Autodesk Inventor part; units mm, degrees
ref_plane "YZ Plane" through (0, 0, 0) normal (1, 0, 0) x (0, 1, 0)
ref_plane "XZ Plane" through (0, 0, 0) normal (0, 1, 0) x (-1, 0, 0)
ref_plane "XY Plane" through (0, 0, 0) normal (0, 0, 1) x (1, 0, 0)
sketch "草圖1" plane through (0, 0, 0) normal (0, 0, 1) x (1, 0, 0)
  circle A0 centre (0, 0) radius 17.5
  circle A1 centre (120, 0) radius 17.5
  line L0 (0, 17.5) -> (120, 17.5)
  line L1 (120, 17.5) -> (120, -17.5)
  line L2 (120, -17.5) -> (0, -17.5)
  line L3 (0, -17.5) -> (0, 17.5)
  dimension "d0" = 35
  dimension "d1" = 35
  dimension "d4" = 120
  dimension "d5" = 35
extrude "擠出1" add sketch "草圖1" along normal blind 15
sketch "草圖2" plane through (0, 0, 15) normal (0, 0, 1) x (1, 0, 0)
  circle A0 centre (0, 0) radius 14
  arc A1 (120, -17.5) -> (120, 17.5) centre (120, 0) ccw
  circle A2 centre (120, 0) radius 14
  dimension "d6" = 28
  dimension "d7" = 28
extrude "擠出2" cut sketch "草圖2" against normal blind 10
sketch "草圖3" plane through (0, 0, 0) normal (1, 0, 0) x (0, 1, 0)
  circle A0 centre (0, -33.7441) radius 48.7441
  point P0 (0, 0)
extrude "擠出3" cut sketch "草圖3" along normal through all both and the other way through all keep common part
sketch "草圖5" plane through (0, 0, 0) normal (0, 0, -1) x (-1, 0, 0)
  circle A0 centre (0, 0) radius 14
  line L0 (0, 17.5) -> (-120, 17.5)
  arc A1 (-120, 17.5) -> (-120, -17.5) centre (-120, 0) ccw
  line L1 (-120, -17.5) -> (0, -17.5)
  arc A2 (0, -17.5) -> (0, 17.5) centre (0, 0) ccw
  line L2 (0, 17.5) -> (-120, 17.5)
  line L3 (-87.5, 17.5) -> (-87.5, -17.5)
  line L4 (-120, -17.5) -> (0, -17.5)
  dimension "d13" = 50
extrude "擠出4" add sketch "草圖5" along normal blind 20 contours A0 | A2 L1 L3 L0
properties part number "第一臂"
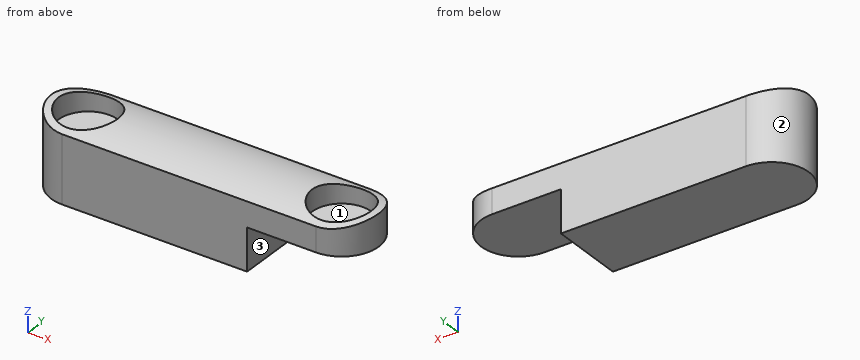
Design review of the part built by this model. Coordinates are the model's own, in mm. Face numbers are marked on the shaded views. A direction names the side the tool comes from. Round coordinates to 2 decimals unless told otherwise and drop trailing zeros. Write each loop counter-clockwise with the first axis right and the second up, starting at its lowest first coordinate (ties: lowest second). Pieces come first, ordered by that corner, then holes.
Item 1: Consider section C-C on x = 113. Give the boundary of the cut face in (y, z).
Item 2: Consider section A-A on z = 7.5. Give the boundary of the cut face in (x, y).
Item 3: For the marked faces 1, 2 and 3, list the 3-axis set-ups (+Z, -Z, +X, -X, +Y, -Y) from which the entire face can be reached by the end or side of a thin tool; tool diameter is ignored.
Item 4: For pin 1 Ø17.5 at (x, y) = (116.5, -3.5) entering from -Z; pin 2 Ø10 at (y, z) = (-7.5, -8) entering from +X; pin 3 Ø3 at (y, z) = (7, 8.5) entering from +X, all flat-tipped, find the tip position at first contact; note any pin that passes through.
Item 5: Consider section D-D on z = -15. Give the boundary of the cut face in (x, y).
Item 6: Consider section B-B on y = 11.5. Give the boundary of the cut face in (x, z).
Item 7: Wall thickness on L1, parallel to X at y = 0, z = 13; L2, parallel to Y at x = 120, z = 10.75; L3, parallel to Z at x = -6, y = 8: over which ranges is each line inside the solid? List them lowest first.
Check values:
1. outline: (-17.5, 0) - (17.5, 0) - (17.5, 11.75) arc R48.74 ccw to (12.12, 13.47) - (12.12, 5) - (-12.12, 5) - (-12.12, 13.47) arc R48.74 ccw to (-17.5, 11.75) - close
2. outline: (0, -17.5) - (120, -17.5) arc R17.5 ccw to (120, 17.5) - (0, 17.5) arc R17.5 ccw to start; hole circle Ø28 at (0, 0); hole circle Ø28 at (120, 0)
3. face 1: +Z
3. face 2: +Z, -Z, -X
3. face 3: -Z, +X, +Y, -Y
4. pin 1: stops at z = 0
4. pin 2: stops at x = 87.5
4. pin 3: stops at x = 136.61
5. outline: (0, -17.5) - (87.5, -17.5) - (87.5, 17.5) - (0, 17.5) arc R17.5 ccw to start
6. outline: (-13.19, -20) - (87.5, -20) - (87.5, 0) - (133.19, 0) - (133.19, 13.62) - (127.98, 13.62) - (127.98, 5) - (112.02, 5) - (112.02, 13.62) - (7.98, 13.62) - (7.98, 5) - (-7.98, 5) - (-7.98, 13.62) - (-13.19, 13.62) - close
7. L1: x = -17.5 to -14, 14 to 106, 134 to 137.5
7. L2: y = -17.5 to -14, 14 to 17.5
7. L3: z = -20 to 5
